Answer from the drawing. Dimensions are ordinates in mm from the lowest x, y and z of the part. A direction names the side the tool comes from. Give positions to 0.01 mm unless a question says otherwise; leave off trailing zeros. Loops run counter-clockwise (first coordinate to the right, second up) from the corner with the lowest first, then second, coordinate; pieces in that order, holes last. Notation, with made-up numbers: (71, 57) -> (121, 57) arc R37 cw to (121, 95) -> close; hole circle Ø2 at (69, 67). An arc over 180 degrees is marked (long way). Return JSON: item names as keys, results as strings. Group by question number.
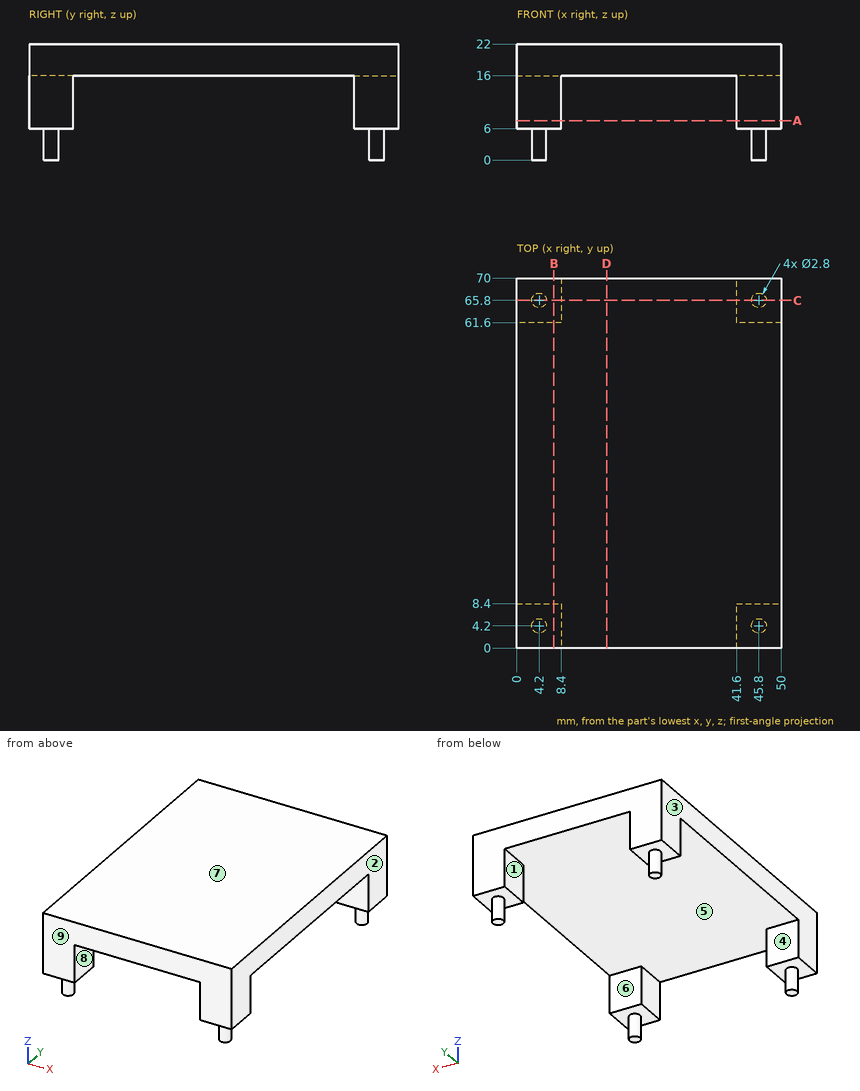
1. Determine the mould class of the marked faces 1, 2, 3 and 4 for opening direction X: pulls with the +X half, pulls with the -X half, needs draft (parallel to the pull), parting line crosses it, or undercut.
2. Section C-C on y = 65.8 is taken. Determine the outline of the cut face in (x, z), then the cut area to 3 significant figures.
3. Section D-D on x = 17 is taken. Determine the outline of the cut face in (y, z).
4. Which of the six approach directions +Z, -Z, +X, -X, +Y, -Y give full straight-line access (tool end or side, diameter ignored) to the marked faces 5, 6, 7, 8 and 9?
5. Section A-A on z = 7.5 is taken. Determine the outline of the cut face in (x, y), then the cut area to 3 significant figures.
6. Section B-B on x = 7 is taken. Determine the outline of the cut face in (y, z), then the cut area to 3 significant figures.
7. Straight lines are drawn through the part: line 1 (Y direction, x = 42.5, z = 11); line 2 (Z direction, x = 43, y = 33). For each, find the intervals that lie inside material, in ascending order. Write a range as from..to.
8. A flat-ended cylindrical pin translates along its axis: pin 1 Ø25 at (x, y) = (36.5, 37) entering from -Z. Find the tip coordinate at first contact, or state that the pin passes through.
Completed:
{
 "1": {"face 1": "undercut", "face 2": "pulls with the +X half", "face 3": "pulls with the -X half", "face 4": "needs draft"},
 "2": {"outline": "(0, 6) -> (2.8, 6) -> (2.8, 0) -> (5.6, 0) -> (5.6, 6) -> (8.4, 6) -> (8.4, 16) -> (41.6, 16) -> (41.6, 6) -> (44.4, 6) -> (44.4, 0) -> (47.2, 0) -> (47.2, 6) -> (50, 6) -> (50, 22) -> (0, 22) -> close", "area": "502 mm²"},
 "3": {"outline": "(0, 16) -> (70, 16) -> (70, 22) -> (0, 22) -> close"},
 "4": {"face 5": "-Z", "face 6": "-Z, +X, -X", "face 7": "+Z, +X, -X, +Y, -Y", "face 8": "-Z, +Y, -Y", "face 9": "+Z, -Z, +X, -X, -Y"},
 "5": {"outline": "(0, 0) -> (8.4, 0) -> (8.4, 8.4) -> (0, 8.4) -> close; (0, 61.6) -> (8.4, 61.6) -> (8.4, 70) -> (0, 70) -> close; (41.6, 0) -> (50, 0) -> (50, 8.4) -> (41.6, 8.4) -> close; (41.6, 61.6) -> (50, 61.6) -> (50, 70) -> (41.6, 70) -> close", "area": "282 mm²"},
 "6": {"outline": "(0, 6) -> (8.4, 6) -> (8.4, 16) -> (61.6, 16) -> (61.6, 6) -> (70, 6) -> (70, 22) -> (0, 22) -> close", "area": "588 mm²"},
 "7": {"line 1": "y = 0..8.4, 61.6..70", "line 2": "z = 16..22"},
 "8": {"pin 1": "stops at z = 16"}
}
